from build123d import *


with BuildPart() as part:
    # 草图1 → 旋转1 (revolve)
    with BuildSketch(Plane.XY, mode=Mode.PRIVATE) as revolve_1_sk:
        Polygon((-21, 0), (-21, 14.8), (-22.83, 16.669359971), (-16.56, 23.56), (-12.34, 16.5), (-0.74246212, 16.5), (0, 15.75753788), (0, 0), align=None)
    revolve(revolve_1_sk.sketch.rotate(Axis((0, 0, 0), (-1, 0, 0)), 270), axis=Axis((0, 0, 0), (-1, 0, 0)))

    # 草图2 → 切除-旋转1 (revolve, cut)
    with BuildSketch(Plane.XY, mode=Mode.PRIVATE) as cut_revolve_1_sk:
        Polygon((-21, 0), (-21, 6.99), (-20.01, 6), (-0.99, 6), (0, 6.99), (0, 0), align=None)
    revolve(cut_revolve_1_sk.sketch.rotate(Axis((0, 0, 0), (-1, 0, 0)), 270), axis=Axis((0, 0, 0), (-1, 0, 0)), mode=Mode.SUBTRACT)


solid = part.part
Can you work these out from the model? Positions are in its coordinate system, mm. A direction names the side the tool comes from. Give positions to 0.01 mm unless a question says otherwise; leave off trailing zeros. Order: outer loops, then holes, each group sorted by start corner. A loop starts at its lowest first (then second) coordinate and runs counter-clockwise, first axis right, second up. Notation, with made-up numbers: (-22, 88.25) - (-17, 88.25) arc R30 ccw to (-17, 124.25) - close; hole circle Ø10 at (37.5, 71.25). An arc over 180 degrees is marked (long way). Write each question's results on one line, items separated by ' | '.
1) I'm going to push flat-ended pins straight in: pin 1 Ø4 at (y, z) = (-3, 8) entering from +X; pin 2 Ø19 at (y, z) = (0, 0) entering from -X; pin 3 Ø1 at (y, z) = (-17, -18) entering from +X; pin 4 Ø1 at (x, z) = (-11, 7.5) entering from -Y. Where does each tip first touch, or does it pass through?
Final values:
pin 1: stops at x = 0 | pin 2: stops at x = -21 | pin 3: passes through | pin 4: stops at y = -14.94
2) Please list where these lines run through material, in increasing order: line 1 along Y through (x, z) = (-8, 0); line 2 along Y through (x, z) = (-21.5, -10.5); line 3 along X through (y, z) = (-7, 5). Write a range as [from, to].
Final values:
line 1: y = [-16.5, -6], [6, 16.5] | line 2: y = [-14.78, -11.14], [11.14, 14.78] | line 3: x = [-21, 0]
3) Suppose I cut it at D-D, the plane x = -19.25. Write out the boundary of the cut face in (y, z).
Final values:
outline: circle Ø41.21 at (0, 0); hole circle Ø12 at (0, 0)
4) Suppose I cut it at C-C, the plane x = -2.5. Write out the boundary of the cut face in (y, z).
Final values:
outline: circle Ø33 at (0, 0); hole circle Ø12 at (0, 0)
5) Suppose I cut it at A-A, the plane y = 0. Write out the boundary of the cut face in (x, z), then the cut area to 3 significant figures.
Final values:
outline: (-22.83, -16.67) - (-16.56, -23.56) - (-12.34, -16.5) - (-0.74, -16.5) - (0, -15.76) - (0, -6.99) - (-0.99, -6) - (-20.01, -6) - (-21, -6.99) - (-21, -14.8) - close; (-22.83, 16.67) - (-21, 14.8) - (-21, 6.99) - (-20.01, 6) - (-0.99, 6) - (0, 6.99) - (0, 15.76) - (-0.74, 16.5) - (-12.34, 16.5) - (-16.56, 23.56) - close | area: 516 mm^2
6) If we mould it in two halves opening along Z, with no side actions, what happens to faces 3 (the face through (-21, 3.5, -6.4)), 4 (the face through (0, -3, 7)), 5 (the face through (-22.44, 5.14, 16.31))? For each: pulls with the +Z half, pulls with the -Z half, needs draft (parallel to the pull), parting line crosses it, or undercut.
Final values:
face 3: undercut | face 4: needs draft | face 5: parting line crosses it
7) On a 3-axis mill with a long thin cutter (end or side, diameter ignored), from which of +Z, -Z, +X, -X, +Y, -Y can I reach the whole of each face in a straight line? I mean faces 1 (the face through (-6.46, -16.108, -3.577)), 2 (the face through (-10.367, 1.802, 5.723)). Say none if no direction works.
Final values:
face 1: +X | face 2: +X, -X
